```python
from build123d import *

# Parameters (mm, degrees)
F1_DEPTH = 25.4
F3_DEPTH = 25.4
F5_DEPTH = 25.4


with BuildPart() as f1:
    # F0 (on Front) → F1 (new body)
    with BuildSketch(Plane.XZ):
        Polygon((-18.4541802113, -5.9961266285), (-29.8594908165, -41.0980633142), (0, -19.4038733715), align=None)
        Polygon((-11.4053106051, 15.6980633142), (-48.3136710278, 15.6980633142), (-18.4541802113, -5.9961266285), align=None)
        Polygon((18.4541802113, -5.9961266285), (11.4053106051, 15.6980633142), (-11.4053106051, 15.6980633142), (-18.4541802113, -5.9961266285), (0, -19.4038733715), align=None)
        Polygon((11.4053106051, 15.6980633142), (0, 50.8), (-11.4053106051, 15.6980633142), align=None)
        Polygon((18.4541802113, -5.9961266285), (48.3136710278, 15.6980633142), (11.4053106051, 15.6980633142), align=None)
        Polygon((0, -19.4038733715), (29.8594908165, -41.0980633142), (18.4541802113, -5.9961266285), align=None)
    extrude(amount=F1_DEPTH)

    # F2 (on face) → F3 (join)
    with BuildSketch(Plane(origin=(0, 0, 0), x_dir=(-1, 0, 0), z_dir=(0, 1, 0))):
        Polygon((-11.4053106051, 15.6980633142), (-18.4541802113, -5.9961266285), (0, -19.4038733715), (18.4541802113, -5.9961266285), (11.4053106051, 15.6980633142), align=None)
    extrude(amount=F3_DEPTH)

    # F4 (on face) → F5 (join)
    with BuildSketch(Plane(origin=(0, 25.4, 0), x_dir=(-1, 0, 0), z_dir=(0, 1, 0))):
        Polygon((7.0488696062, 2.2903165712), (4.3564409989, -5.9961266285), (18.4541802113, -5.9961266285), align=None)
        Polygon((11.4053106051, 15.6980633142), (0, 7.4116201145), (7.0488696062, 2.2903165712), align=None)
        Polygon((0, 7.4116201145), (-7.0488696062, 2.2903165712), (-4.3564409989, -5.9961266285), (4.3564409989, -5.9961266285), (7.0488696062, 2.2903165712), align=None)
        Polygon((-11.4053106051, 15.6980633142), (-7.0488696062, 2.2903165712), (0, 7.4116201145), align=None)
        Polygon((-7.0488696062, 2.2903165712), (-18.4541802113, -5.9961266285), (-4.3564409989, -5.9961266285), align=None)
        Polygon((4.3564409989, -5.9961266285), (-4.3564409989, -5.9961266285), (0, -19.4038733715), align=None)
    extrude(amount=F5_DEPTH)


solid = f1.part
```
Model file for the job. Use its own axes, mm. A direction names the side the tool comes from. Coordinates: 2 decimals unless noted, no trailing zeros. Write each loop counter-clockwise with the first axis right and the second up, starting at its lowest first coordinate (ties: lowest second). Pieces come first, ordered by that corner, then holes. Notation, with made-up numbers: (-20.5, 24.5) - (-16.5, 24.5) arc R27 cw to (-16.5, 51.5) - close; hole circle Ø6 at (13, 85). An arc over 180 degrees is marked (long way). One line per item, written item: value. Start each with the question number.
1. Flat gauge pins, fed straight in: pin 1 (3 mm diameter, centred on y = 6.5, z = 5.5, fed in from -X); pin 2 (4 mm diameter, centred on y = 13.5, z = -12, fed in from -X); pin 3 (2 mm diameter, centred on y = -6, z = 2, fed in from +X). Where does each tip first touch, or does it go through?
2. Slice it at B-B (y = 9). Write the cut outline in (x, z).
3. Mould opens along X. For faces 1 (the flat face through (14.72, -12.52, -30.1)), 2 (the flat face through (9.26, 37.92, 9.09)), 3 (the flat face through (13, 25.4, 5)) say: released by +X, released by -X, zero draft, split by the parting line, or undercut.
4. Slice it at A-A (z = -25). Write the cut outline in (x, y), plus the area to 3 significant figures.
5. Slice it at D-D (y = -4). Write the cut outline in (x, z).
6. Probe line 1 (Y direction, x = -6, z = -23); line 2 (X direction, y = 22.5, z = 5); line 3 (Z direction, x = -4.5, y = 35). List the from-to ranges inside material, lowest first. Write a range as from..to.
7. Tool access for faces 4 (the flat face through (-5.78, 37.92, 11.61)), 5 (the flat face through (-15, 0, -23)), 6 (the flat face through (-13, 25.4, 5)): list every direction of +Z, -Z, +X, -X, +Y, -Y with a clear straight run to the whole face (end or side of a thin tool).
8. Slice it at C-C (x = -2.5). Write the cut outline in (y, z), plus the area to 3 significant figures.
Answers below:
1. pin 1: stops at x = -15.21
1. pin 2: stops at x = -12.94
1. pin 3: stops at x = 30.84
2. outline: (-18.45, -6) - (0, -19.4) - (18.45, -6) - (11.41, 15.7) - (-11.41, 15.7) - close
3. face 1: undercut
3. face 2: released by +X
3. face 3: zero draft
4. outline: (-24.63, -25.4) - (-7.7, -25.4) - (-7.7, 0) - (-24.63, 0) - close; (7.7, -25.4) - (24.63, -25.4) - (24.63, 0) - (7.7, 0) - close
4. area: 860 mm^2
5. outline: (-48.31, 15.7) - (-18.45, -6) - (-29.86, -41.1) - (0, -19.4) - (29.86, -41.1) - (18.45, -6) - (48.31, 15.7) - (11.41, 15.7) - (0, 50.8) - (-11.41, 15.7) - close
6. line 1: y = -25.4..0
6. line 2: x = -14.88..14.88
6. line 3: z = -6..10.68
7. face 4: +Z, +Y
7. face 5: -Z, -X, +Y
7. face 6: -X, +Y
8. outline: (-25.4, -21.22) - (0, -21.22) - (0, -17.59) - (25.4, -17.59) - (25.4, -11.71) - (50.8, -11.71) - (50.8, 9.23) - (25.4, 9.23) - (25.4, 15.7) - (0, 15.7) - (0, 43.11) - (-25.4, 43.11) - close
8. area: 3,010 mm^2
